CAD build for the part. Positions are in the model's coordinates, mm. Face numbers are marked on the shaded views. A direction names the side the tool comes from. Coordinates: 2 decimals unless noted, no trailing zeros. Loops run counter-clockwise (first coordinate to the right, second up) from the corner with the lowest first, then second, coordinate; pieces in that order, holes last. Notation, with made-up numbers: (0, 88.5) -> (38, 88.5) arc R17 cw to (38, 105.5) -> close; hole circle Ø8 at (36.5, -11). An arc over 180 degrees is marked (long way). Write each question's results on one line, items separated by ' | '.
from build123d import *

# Parameters (mm, degrees)
F0_R     = 25.308413
F0_R_2   = 7.5
F1_DEPTH = 10
F2_T     = -1.5


with BuildPart() as f1:
    # F0 (on Top) → F1 (new body)
    with BuildSketch(Plane.XY):
        Circle(F0_R)
        with Locations((0, -13.165262)):
            Circle(F0_R_2, mode=Mode.SUBTRACT)
        with Locations((0, 11.95744)):
            Circle(F0_R_2, mode=Mode.SUBTRACT)
    extrude(amount=F1_DEPTH)

    # F2
    f2_openings = [f1.faces().sort_by_distance(p)[0] for p in [
        (0, 0.12867, 0),
    ]]
    offset(amount=F2_T, openings=f2_openings)


solid = f1.part
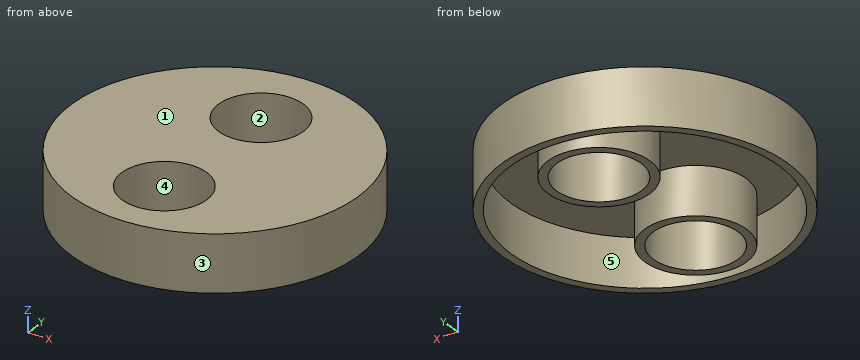
1) Pin check, flat tips, straight feed: pin 1 (3 mm diameter, centred on x = -6.5, z = 8.5, fed in from +Y); pin 2 (2 mm diameter, centred on x = 0.5, z = 4.5, fed in from -Y); pin 3 (4 mm diameter, centred on x = 14.5, z = 5.5, fed in from +Y). Stop position of each tip, or through.
Outcome:
pin 1: stops at y = 24.81 | pin 2: stops at y = -25.31 | pin 3: stops at y = 22.01
2) Slice it at D-D (y = 0). Write the cut outline in (x, z), then the cut area to 3 significant figures.
Outcome:
outline: (-25.31, 0) -> (-23.81, 0) -> (-23.81, 8.5) -> (23.81, 8.5) -> (23.81, 0) -> (25.31, 0) -> (25.31, 10) -> (-25.31, 10) -> close | area: 101 mm^2
3) Two-plate mould, pull along X, no slides. Class the marked faces 1, 2 and 3: pulls with the +X half, pulls with the -X half, needs draft (parallel to the pull), parting line crosses it, or undercut.
Outcome:
face 1: needs draft | face 2: undercut | face 3: parting line crosses it
4) Slice it at A-A (z = 6.5). Write the cut outline in (x, y).
Outcome:
outline: circle Ø50.62 at (0, 0); circle Ø18 at (0, -13.17); circle Ø18 at (0, 11.96); hole circle Ø47.62 at (0, 0); hole circle Ø15 at (0, -13.17); hole circle Ø15 at (0, 11.96)
5) Which spindle directions (+Z, -Z, +X, -X, +Y, -Y) get a long thin tool onto all of the face, cutting with end or side? Do the marked faces 4 and 5. Say none if no direction does.
Outcome:
face 4: +Z, -Z | face 5: -Z
6) Slice it at B-B (x = 0). Write the cut outline in (y, z).
Outcome:
outline: (-25.31, 0) -> (-23.81, 0) -> (-23.81, 8.5) -> (-22.17, 8.5) -> (-22.17, 0) -> (-20.67, 0) -> (-20.67, 10) -> (-25.31, 10) -> close; (-5.67, 0) -> (-4.17, 0) -> (-4.17, 8.5) -> (2.96, 8.5) -> (2.96, 0) -> (4.46, 0) -> (4.46, 10) -> (-5.67, 10) -> close; (19.46, 0) -> (20.96, 0) -> (20.96, 8.5) -> (23.81, 8.5) -> (23.81, 0) -> (25.31, 0) -> (25.31, 10) -> (19.46, 10) -> close
7) Slice it at C-C (y = 5.5). Write the cut outline in (x, z), then the cut area to 3 significant figures.
Outcome:
outline: (-24.7, 0) -> (-23.16, 0) -> (-23.16, 8.5) -> (-6.27, 8.5) -> (-6.27, 0) -> (-3.81, 0) -> (-3.81, 10) -> (-24.7, 10) -> close; (3.81, 0) -> (6.27, 0) -> (6.27, 8.5) -> (23.16, 8.5) -> (23.16, 0) -> (24.7, 0) -> (24.7, 10) -> (3.81, 10) -> close | area: 131 mm^2
8) Drill centre lines: L1, parallel to Y at x = 0, z = 2.5; L2, parallel to X at y = 5, z = 2; L3, parallel to Y at x = 2.5, z = 6.75. Where is each one in solid material? Low to high. Write a range as from..to.
Outcome:
L1: y = -25.31..-23.81, -22.17..-20.67, -5.67..-4.17, 2.96..4.46, 19.46..20.96, 23.81..25.31 | L2: x = -24.81..-23.28, -5.71..-2.8, 2.8..5.71, 23.28..24.81 | L3: y = -25.18..-23.68, -21.81..-20.24, -6.09..-4.52, 3.31..4.89, 19.03..20.6, 23.68..25.18
